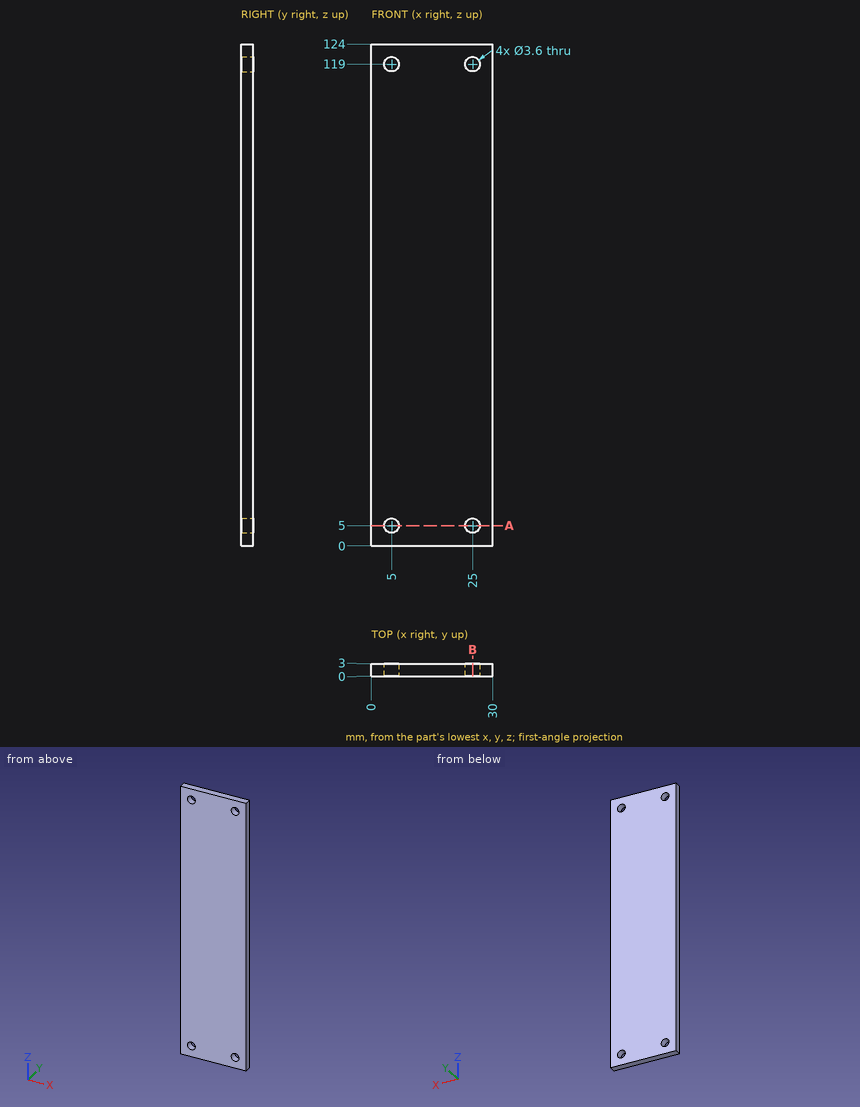
For this review, use the dimensioned drawing (mm, ordinates from the lowest corner) and the shaded views. Coordinates: 2 decimals unless noted, no trailing zeros. Write each loop counter-clockwise with the first axis right and the second up, starting at its lowest first coordinate (ties: lowest second). Pieces come first, ordered by that corner, then holes. Notation, with made-up numbers: (7, 77.5) -> (66, 77.5) arc R15 cw to (66, 89.5) -> close; hole circle Ø10 at (68.25, 65). An arc over 180 degrees is marked (long way). Put each result on its own line as item: value.
Q1. Take a section at B-B, the plane x = 25. State the section outline as (y, z) points.
From the geometry:
outline: (0, 0) -> (3, 0) -> (3, 3.2) -> (0, 3.2) -> close; (0, 6.8) -> (3, 6.8) -> (3, 117.2) -> (0, 117.2) -> close; (0, 120.8) -> (3, 120.8) -> (3, 124) -> (0, 124) -> close
Q2. Wall thickness on L1, parallel to X at y = 0.85, z = 119; L2, parallel to Z at x = 25, y = 0.4; L3, parallel to Z at x = 5.75, y = 0.35: over which ranges is each line inside the solid? List them lowest first.
From the geometry:
L1: x = 0 to 3.2, 6.8 to 23.2, 26.8 to 30
L2: z = 0 to 3.2, 6.8 to 117.2, 120.8 to 124
L3: z = 0 to 3.36, 6.64 to 117.36, 120.64 to 124
Q3. Clearance check with a flat-ended pin moving along its axis: pin 1 Ø2 at (x, z) = (25, 5) entering from -Y. State where the tip first meets the part, or that it passes through.
From the geometry:
pin 1: passes through
Q4. Take a section at A-A, the plane z = 5. State the section outline as (x, y) points, then the cut area to 3 significant figures.
From the geometry:
outline: (0, 0) -> (3.2, 0) -> (3.2, 3) -> (0, 3) -> close; (6.8, 0) -> (23.2, 0) -> (23.2, 3) -> (6.8, 3) -> close; (26.8, 0) -> (30, 0) -> (30, 3) -> (26.8, 3) -> close
area: 68.4 mm2
